Verification items for the finished model (mm, model axes). A direction names the side the tool comes from. Give positions to 0.01 mm unless a question says otherwise; leave off trailing zeros. Order: outer loops, then holes, each group sorted by start corner. A loop starts at its lowest first (then second) coordinate and runs counter-clockwise, first axis right, second up. Notation, with made-up numbers: M 33.25,36.5 L 41.25,36.5 A19 cw 41.25,66.5 Z; hole C -39.5,9.25 d1. An arc over 180 degrees is marked long. Answer as a JSON object with one key per item and string values.
Autodesk Inventor part; units mm, degrees
ref_plane "YZ Plane" through (0, 0, 0) normal (1, 0, 0) x (0, 1, 0)
ref_plane "XZ Plane" through (0, 0, 0) normal (0, 1, 0) x (-1, 0, 0)
ref_plane "XY Plane" through (0, 0, 0) normal (0, 0, 1) x (1, 0, 0)
sketch "Sketch3" plane through (0, 0, 0) normal (0, 1, 0) x (-1, 0, 0)
  line L0 (2.7739, 2.9) -> (-22.6261, 2.9)
  line L1 (-22.6261, 2.9) -> (-22.6261, -22.5)
  line L2 (-22.6261, -22.5) -> (2.7739, -22.5)
  line L3 (2.7739, -22.5) -> (2.7739, 2.9)
  line L4 (-22.6261, 2.9) -> (-21.0386, 2.9)
  line L5 (-21.0386, -20.9125) -> (1.1864, -20.9125)
  line L6 (1.1864, -20.9125) -> (1.1864, 1.3125)
  line L7 (1.1864, 1.3125) -> (-21.0386, 1.3125)
  line L8 (-21.0386, 1.3125) -> (-21.0386, -20.9125)
  point P0 (0, 0)
  dimension "d4" = 25.4
  dimension "d5" = 25.4
  dimension "d6" = 1.5875
  dimension "d7" = 23.8125
  dimension "d8" = 22.225
  dimension "d9" = 22.225
extrude "Extrusion2" add sketch "Sketch3" along normal blind 38.1
sketch "Sketch5" plane through (-2.7739, 0, 2.9) normal (0, 0, 1) x (1, 0, 0)
  line L0 (0, 38.1) -> (25.4, 38.1)
  circle A0 centre (12.7, 38.1) radius 12.7
  point P0 (2.7739, 0)
extrude "Extrusion4" cut sketch "Sketch5" against normal blind 25.4
sketch "Sketch8" plane through (-2.7739, 0, -22.5) normal (-1, 0, 0) x (0, 0, 1)
  circle A0 centre (12.7, 12.7079) radius 3.9751
  point P0 (22.5, 0)
  dimension "d22" = 7.9502
extrude "Extrusion6" cut sketch "Sketch8" against normal blind 12.7
properties part number "Seat tab to frame mount"
Q1. Section check A-A on y = 24. Record the cut outline in (x, z).
Resolved:
{"outline": "M -2.77,-22.5 L 22.63,-22.5 L 22.63,2.9 L -2.77,2.9 Z; hole M -1.19,-20.91 L 21.04,-20.91 L 21.04,1.31 L -1.19,1.31 Z"}
Q2. Release check for a two-part mould opening along Z. For faces 3 (the face through (10, 15, 2.9)), 4 (the face through (-1.991, 11.185, -6.128)), 5 (the face through (21.3, 0, -9.7)), 6 (the face through (10, 15, -22.5)) record: +Z half, -Z half, draft (parallel to the pull), parting line (faces both ways), or undercut.
Resolved:
{"face 3": "+Z half", "face 4": "undercut", "face 5": "draft", "face 6": "-Z half"}
Q3. Gauge pin test, flat end, axial feed: pin 1 Ø4 at (x, z) = (10.5, -0.5) entering from +Y. Record the tip position at first contact, or that the pin passes through.
Resolved:
{"pin 1": "stops at y = 25.48"}
Q4. Section check D-D on x = 19. Record the cut outline in (y, z).
Resolved:
{"outline": "M 0,-22.5 L 29.21,-22.5 L 29.21,-20.91 L 0,-20.91 Z; M 0,1.31 L 29.21,1.31 L 29.21,2.9 L 0,2.9 Z"}
Q5. Section check C-C on z = -9.8. Record the cut outline in (x, y).
Resolved:
{"outline": "M -2.77,0 L -1.19,0 L -1.19,8.73 L -2.77,8.73 Z; M -2.77,16.68 L -1.19,16.68 L -1.19,31.95 A12.7 cw -2.77,38.1 Z; M 21.04,0 L 22.63,0 L 22.63,38.1 A12.7 cw 21.04,31.95 Z"}
Q6. Tool access check on faces 1 (the face through (-2.774, 19, -10)), 2 (the face through (10, 12, -20.912)). Record the directions out of +Z, -Z, +X, -X, +Y, -Y that give a thin tool (end or side, any length) a straight path to the whole face; none if there is none.
Resolved:
{"face 1": "+Z, -Z, -X, +Y, -Y", "face 2": "+Y, -Y"}
Q7. Section check B-B on z = -16. Record the cut outline in (x, y), then the cut area to 3 significant figures.
Resolved:
{"outline": "M -2.77,0 L -1.19,0 L -1.19,31.95 A12.7 cw -2.77,38.1 Z; M 21.04,0 L 22.63,0 L 22.63,38.1 A12.7 cw 21.04,31.95 Z", "area": "108 mm²"}
Q8. Material ranges on L1, parallel to Z at x = 1.25, y = 3; L2, parallel to X at y = 19.5, z = -0.25; L3, parallel to Y at x = -1.75, z = -9.8, recorded low to high.
Resolved:
{"L1": "z = -22.5 to -20.91, 1.31 to 2.9", "L2": "x = -2.77 to -1.19, 21.04 to 22.63", "L3": "y = 0 to 8.73, 16.68 to 33.1"}
